Autodesk Inventor part; units mm, degrees
ref_plane "YZ Plane" through (0, 0, 0) normal (1, 0, 0) x (0, 1, 0)
ref_plane "XZ Plane" through (0, 0, 0) normal (0, 1, 0) x (-1, 0, 0)
ref_plane "XY Plane" through (0, 0, 0) normal (0, 0, 1) x (1, 0, 0)
sketch "Sketch1" plane through (0, 0, 0) normal (1, 0, 0) x (0, 1, 0)
  line L0 (0, 0) -> (0, -152.4)
  line L1 (0, -152.4) -> (25.4, -152.4)
  line L2 (25.4, -152.4) -> (25.4, -114.3)
  line L3 (25.4, -114.3) -> (63.5, -114.3)
  line L4 (63.5, -114.3) -> (63.5, -152.4)
  line L5 (63.5, -152.4) -> (88.9, -152.4)
  line L6 (88.9, -152.4) -> (88.9, -88.9)
  line L7 (0, 0) -> (88.9, 0)
  line L8 (88.9, 0) -> (88.9, -38.1)
  line L9 (88.9, -38.1) -> (44.45, -38.1)
  line L10 (44.45, -38.1) -> (88.9, -88.9)
  dimension "d0" = 152.4
extrude "Extrusion1" add sketch "Sketch1" along normal blind 25.4
properties part number "P2-1"
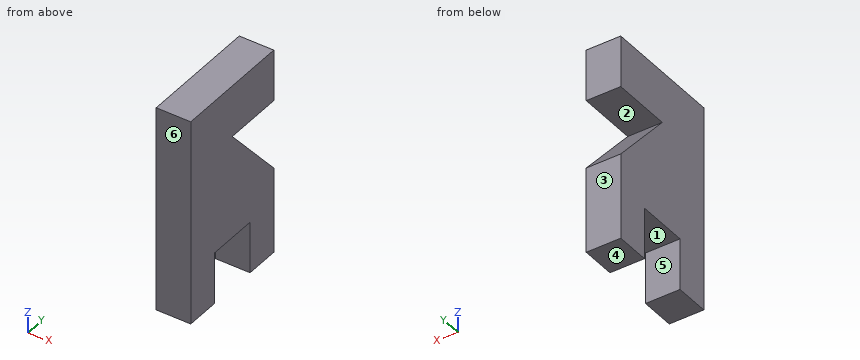
Design review of the part built by this model. Coordinates are the model's own, in mm. Face numbers are marked on the shaded views. A direction names the side the tool comes from. Coordinates: 2 decimals unless noted, no trailing zeros. Order: outer loops, then holes, each group sorted by start corner. A loop starts at its lowest first (then second) coordinate and runs counter-clockwise, first axis right, second up. Notation, with made-up numbers: (89, 89.25) - (139, 89.25) arc R14 cw to (139, 115.25) - close; hole circle Ø2 at (12.25, 81.5). An arc over 180 degrees is marked (long way). Put each result on its own line as item: value.
1) The part is to be moulded in two halves that separate along Y. For the marked faces 4, 5 and 6, say which applies: released by +Y, released by -Y, zero draft, split by the parting line, or undercut.
Response values:
face 4: zero draft
face 5: undercut
face 6: released by -Y
2) Tool access review of the marked faces 1, 2 and 3: name each direction out of +Z, -Z, +X, -X, +Y, -Y from which nothing blocks a thin tool from reaching the whole face with its end or side.
Response values:
face 1: -Z, +X, -X
face 2: +X, -X, +Y
face 3: +Z, -Z, +X, -X, +Y
3) Take a section at D-D, the plane z = -68.5. Give the boundary of the cut face in (x, y).
Response values:
outline: (0, 0) - (25.4, 0) - (25.4, 71.05) - (0, 71.05) - close
4) Take a section at A-A, the plane z = -120.5. Give the boundary of the cut face in (x, y).
Response values:
outline: (0, 0) - (25.4, 0) - (25.4, 25.4) - (0, 25.4) - close; (0, 63.5) - (25.4, 63.5) - (25.4, 88.9) - (0, 88.9) - close
5) Insertion check: P1, Ø7.5, axis at x = 17, y = 36, coming from the -Z side; P2, Ø2, axis at x = 17, y = 62, coming from the +Z side; P3, Ø1, axis at x = 22.5, z = -42.5, coming from the +Y side. Each pin has a flat end and moves straight along its axis. Give the tip position at first contact, or say it passes through.
Response values:
P1: stops at z = -114.3
P2: stops at z = 0
P3: stops at y = 48.74
6) Take a section at C-C, the plane x = 4. Give the boundary of the cut face in (y, z).
Response values:
outline: (0, -152.4) - (25.4, -152.4) - (25.4, -114.3) - (63.5, -114.3) - (63.5, -152.4) - (88.9, -152.4) - (88.9, -88.9) - (44.45, -38.1) - (88.9, -38.1) - (88.9, 0) - (0, 0) - close
7) Wall thickness on L1, parallel to Y at x = 21.5, z = -133.5; L2, parallel to Z at x = 18.75, y = 50; L3, parallel to Z at x = 14.25, y = 64.5: over which ranges is each line inside the solid? List them lowest first. Write a range as from..to.
Response values:
L1: y = 0..25.4, 63.5..88.9
L2: z = -114.3..-44.44, -38.1..0
L3: z = -152.4..-61.01, -38.1..0
8) Take a section at B-B, the plane y = 78. Give the boundary of the cut face in (x, z).
Response values:
outline: (0, -152.4) - (25.4, -152.4) - (25.4, -76.44) - (0, -76.44) - close; (0, -38.1) - (25.4, -38.1) - (25.4, 0) - (0, 0) - close
